Check sheet for the modelled part. Datum: model origin and axes. Units: mm. A direction names the side the tool comes from. Round coordinates to 2 decimals unless told otherwise and drop trailing zeros. Order: outer loops, then holes, each group sorted by start corner. A loop starts at its lowest first (then second) coordinate and runs counter-clockwise, first axis right, second up. Notation, with made-up numbers: (1.5, -32.5) -> (52.5, -32.5) arc R15 cw to (52.5, -16.5) -> close; hole circle Ø10 at (0, 42.25). An arc over 180 degrees is marked (long way). Answer in a Markdown table with one row per item. Add a question column.
1. Material ranges on L1, parallel to Z at x = 4.5, y = 12.5; L2, parallel to Y at x = 5.75, z = 0.25; L3, parallel to X at y = 11.5, z = -2.5, recorded low to high. Write a range as from..to.
2. Sectioned sample at A-A, the plane x = 4. Record the boundary of the cut face in (y, z), then the cut area to 3 significant figures.
3. Sectioned sample at C-C, the plane y = 10.25. Record the boundary of the cut face in (x, z), then the cut area to 3 significant figures.
4. Sectioned sample at D-D, the plane x = 5.75. Record the boundary of the cut face in (y, z).
5. Sectioned sample at B-B, the plane z = 8.25. Record the boundary of the cut face in (x, y), then the cut area to 3 significant figures.
6. Access from +Z, -Z, +X, -X, +Y, -Y to the whole of each face (thin tool, end or side, straight path). Record for faces 5 (the flat face through (3, -2, 20)), 6 (the flat face through (3, 7, 0)).
7. Draft check along X on faces 1 (the flat face through (6.096, 2, -1)), 2 (the cylindrical face through (2.122, 3.363, -2.535)), 3 (the flat face through (3, 0, 10)), 4 (the flat face through (0, 2, -1)). Enter one of: +X half, -X half, draft (parallel to the pull), parting line (faces both ways), or undercut.
8. Depth check by flat-ended pin: P1, Ø3, axis at x = 3, z = 14, coming from the +Y side; P2, Ø6, axis at y = 8.5, z = 0.5, coming from the -X side; P3, Ø2.5, axis at x = 3.05, y = 10.54, coming from the +Z side. Enter the tip coordinate at first touch or a pass-through.
```python
from build123d import *

# Parameters (mm, degrees)
BOSS_EXTRUDE2_DEPTH = 6.096
SKETCH3_R           = 1.524
SKETCH3_R_2         = 1.525
CUT_EXTRUDE1_DEPTH  = 30.380027597
SKETCH4_R           = 1.524
SKETCH4_R_2         = 1.525
CUT_EXTRUDE3_DEPTH  = 26.262343945


with BuildPart() as part:
    # Sketch2 → Boss-Extrude2 (new body)
    with BuildSketch(Plane(origin=(0, 0, 0), x_dir=(0, 0, -1), z_dir=(1, 0, 0))):
        Polygon((0, 0), (0, 14.178321678), (5, 14.178321678), (5, -3), (-20, -3), (-20, 0), align=None)
    extrude(amount=BOSS_EXTRUDE2_DEPTH)

    # Sketch3 → Cut-Extrude1 (cut, through all)
    with BuildSketch(Plane(origin=(0, 0, -5), x_dir=(-1, 0, 0), z_dir=(0, 0, -1))):
        with Locations(Location((-3.05, 10.538720291, 0), (0, 0, 90))):
            Circle(SKETCH3_R)
        with Locations(Location((-3.05, 4.572872866, 0), (0, 0, 90))):
            Circle(SKETCH3_R_2)
    extrude(amount=-CUT_EXTRUDE1_DEPTH, mode=Mode.SUBTRACT)

    # Sketch4 → Cut-Extrude3 (cut, through all)
    with BuildSketch(Plane(origin=(0, 0, 0), x_dir=(1, 0, 0), z_dir=(0, 1, 0))):
        with Locations(Location((3.046, -7.206821765, 0), (0, 0, 270))):
            Circle(SKETCH4_R)
        with Locations(Location((3.046, -13.556821765, 0), (0, 0, 270))):
            Circle(SKETCH4_R_2)
    extrude(amount=-CUT_EXTRUDE3_DEPTH, mode=Mode.SUBTRACT)


solid = part.part
```
Answer key:
| question | item | result |
|---|---|---|
| 1 | L1 | z = -5..0 |
| 1 | L2 | y = -3..0 |
| 1 | L3 | x = 0..1.87, 4.23..6.1 |
| 2 | outline | (-3, -5) -> (3.38, -5) -> (3.38, 0) -> (0, 0) -> (0, 6.02) -> (-3, 6.02) -> close; (-3, 8.4) -> (0, 8.4) -> (0, 12.37) -> (-3, 12.37) -> close; (-3, 14.75) -> (0, 14.75) -> (0, 20) -> (-3, 20) -> close; (5.77, -5) -> (9.35, -5) -> (9.35, 0) -> (5.77, 0) -> close; (11.73, -5) -> (14.18, -5) -> (14.18, 0) -> (11.73, 0) -> close |
| 2 | area | 108 mm² |
| 3 | outline | (0, -5) -> (1.55, -5) -> (1.55, 0) -> (0, 0) -> close; (4.55, -5) -> (6.1, -5) -> (6.1, 0) -> (4.55, 0) -> close |
| 3 | area | 15.5 mm² |
| 4 | outline | (-3, -5) -> (14.18, -5) -> (14.18, 0) -> (0, 0) -> (0, 20) -> (-3, 20) -> close |
| 5 | outline | (0, -3) -> (1.93, -3) -> (1.93, 0) -> (0, 0) -> close; (4.16, -3) -> (6.1, -3) -> (6.1, 0) -> (4.16, 0) -> close |
| 5 | area | 11.6 mm² |
| 6 | face 5 | +Z, +X, -X, +Y, -Y |
| 6 | face 6 | +Z, +X, -X, +Y |
| 7 | face 1 | +X half |
| 7 | face 2 | undercut |
| 7 | face 3 | draft |
| 7 | face 4 | -X half |
| 8 | P1 | stops at y = 0 |
| 8 | P2 | stops at x = 0 |
| 8 | P3 | passes through |
